Part print with two shaded views. Sizes in mm from the minimum x, y, z corner. Coordinates: 2 decimals unless noted, no trailing zeros. Order: outer loops, then holes, each group sorted by start corner. A loop starts at its lowest first (then second) coordinate and runs counter-clockwise, first axis right, second up. Notation, with made-up numbers: (68, 24.25) - (78, 24.25) arc R9 cw to (78, 41.25) - close; hole circle Ø4 at (-36, 76). An arc over 180 degrees is marked (long way). Return JSON: item names as keys, results as strings.
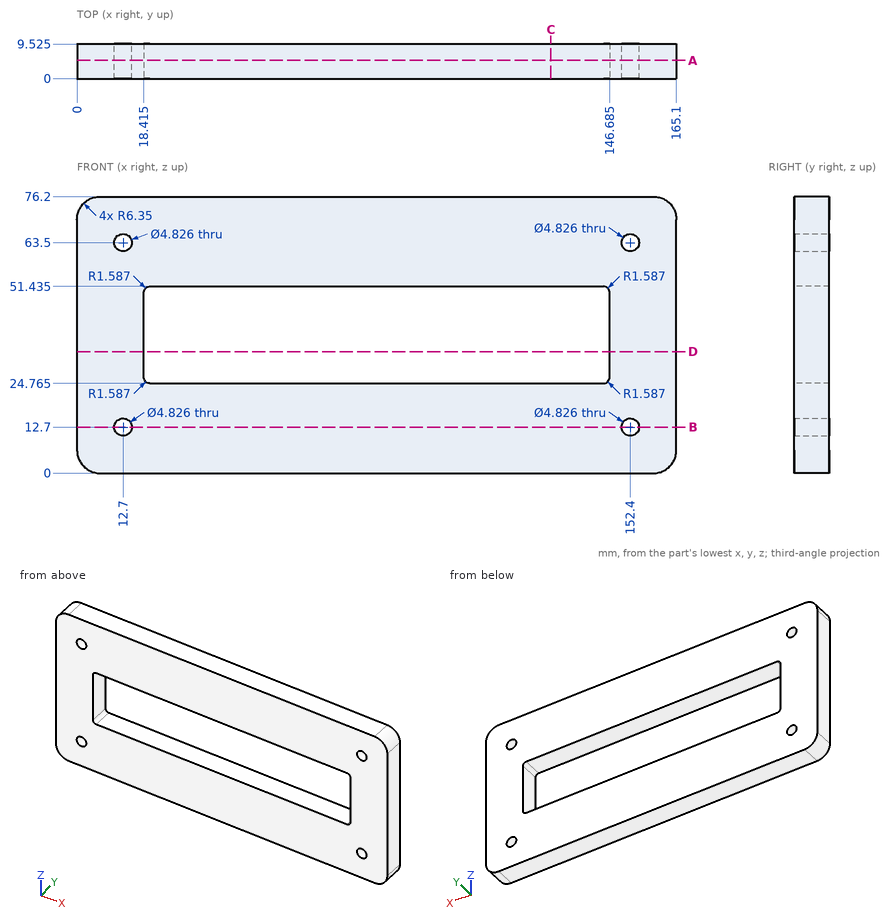
Item 1: Wall check: L1, parallel to Z at x = 12.7, y = 6.5; L2, parallel to Z at x = 59.5, y = 4.5 (1 decimal); L3, parallel to X at y = 3.5, z = 28 (1 decimal). Give the ranges that are in metal, low to high. Write a range as [from, to].
Findings below:
{"L1": "z = [0, 10.29], [15.11, 61.09], [65.91, 76.2]", "L2": "z = [0, 24.8], [51.4, 76.2]", "L3": "x = [0, 18.4], [146.7, 165.1]"}
Item 2: Band-saw the part on D-D, the plane z = 33.5. List the corners of the cut face in (x, y) (1 decimal), then the cut area to 3 significant figures.
Findings below:
{"outline": "(0, 0) - (18.4, 0) - (18.4, 9.5) - (0, 9.5) - close; (146.7, 0) - (165.1, 0) - (165.1, 9.5) - (146.7, 9.5) - close", "area": "351 mm²"}
Item 3: Band-saw the part on A-A, the plane y = 5. Count the separate pieces of the cut face and the enclosed holes in it, then the cut area to 3 significant figures.
Findings below:
{"separate pieces": "1", "enclosed holes": "5", "area": "9,050 mm²"}
Item 4: Band-saw the part on B-B, the plane z = 12.7. List the corners of the cut face in (x, y) (1 decimal), then the cut area to 3 significant figures.
Findings below:
{"outline": "(0, 0) - (10.3, 0) - (10.3, 9.5) - (0, 9.5) - close; (15.1, 0) - (150, 0) - (150, 9.5) - (15.1, 9.5) - close; (154.8, 0) - (165.1, 0) - (165.1, 9.5) - (154.8, 9.5) - close", "area": "1,480 mm²"}
Item 5: Drop a flat-ended pin along its axis: P1, Ø4.5, axis at x = 12.7, z = 63.5, coming from the +Y side. Give the stop position or say it passes through.
Findings below:
{"P1": "passes through"}
Item 6: Band-saw the part on C-C, the plane x = 130.5. List the corners of the cut face in (y, z) (1 decimal), then the cut area to 3 significant figures.
Findings below:
{"outline": "(0, 0) - (9.5, 0) - (9.5, 24.8) - (0, 24.8) - close; (0, 51.4) - (9.5, 51.4) - (9.5, 76.2) - (0, 76.2) - close", "area": "472 mm²"}
